Work out the finished part from the listing and answer in its coordinate system (mm). Face numbers are marked on the shaded views. A direction names the side the tool comes from. Give positions to 0.01 mm unless a question says otherwise; leave off trailing zeros. Loops run counter-clockwise (first coordinate to the right, second up) from the corner with the lowest first, then second, coordinate; pieces in that order, holes last. Notation, with made-up numbers: M 81.5,60 L 138.5,60 A25 cw 138.5,86 Z; hole C 64,8.5 d11. An arc over 180 degrees is marked long. Write item = value, one per line. Start each with the question number.
1. For the marked faces 1 and 2, determine the directions among +Z, -Z, +X, -X, +Y, -Y from which every point of the face is accessible in a straight line to the end or side of a thin tool.
2. Section B-B on z = -4.5 is taken. Determine the outline of the cut face in (x, y) (1 decimal), plus the area to 3 significant figures.
3. Flat-ended cylindrical pins translate along their axes: pin 1 Ø1 at (y, z) = (-2, -10) entering from -X; pin 2 Ø2 at (x, z) = (1, -9.5) entering from -Y; pin 3 Ø2 at (x, z) = (-2.5, -8) entering from -Y. Find the tip coordinate at first contact, or state that the pin passes through.
4. Section C-C on x = 2.75 is taken. Determine the outline of the cut face in (y, z) (3 decimals).
5. Consider L1, parallel to Z at x = 1.5, y = 2.5 (3 decimals); L2, parallel to Y at x = -1, z = -9.75; L3, parallel to Z at x = -0.75, y = -1 (3 decimals). Determine where each line is inside the solid, lowest interval first. Write a range as [from, to].
Solid Edge part; units mm, degrees
sketch "Sketch1" plane through (0, 0, 0) normal (0, 0, 1) x (1, 0, 0)
  circle A0 centre (0, 0) radius 6.4452
extrude "Protrusion1" add sketch "Sketch1" along normal blind 3.175
sketch "Sketch2" plane through (0, 0, 0) normal (0, 0, -1) x (1, 0, 0)
  circle A0 centre (0, 0) radius 2.0828
extrude "Protrusion2" add sketch "Sketch2" along normal blind 12.7
sketch "Sketch3" plane through (0, 0, -12.7) normal (0, 0, -1) x (1, 0, 0)
  circle A0 centre (0, 0) radius 2.0825
extrude "Cutout1" cut sketch "Sketch3" against normal blind 12.6873 flip side to cut
sketch "Sketch4" plane through (0, 0, 3.175) normal (0, 0, 1) x (1, 0, 0)
  line L0 (-5.609, 3.175) -> (5.609, 3.175)
extrude "Cutout2" cut sketch "Sketch4" against normal up to next material side at (0, 3.225, 3.175)
sketch "Sketch5" plane through (0, 0, 0) normal (1, 0, 0) x (0, 1, 0)
  line L0 (-0.7937, -12.7) -> (-2.0825, -10.4677)
revolve "RevolvedCutout1" cut sketch "Sketch5" angle 360 about axis through (0, 0, -14.7796) along (0, 0, 1) material side at (0, -1.4814, -11.6088)
pattern_circular "Pattern1" count 6 over 360 about axis through (0, 0, 3.175) along (0, 0, 1) of "Cutout2"
properties part number "24102273"
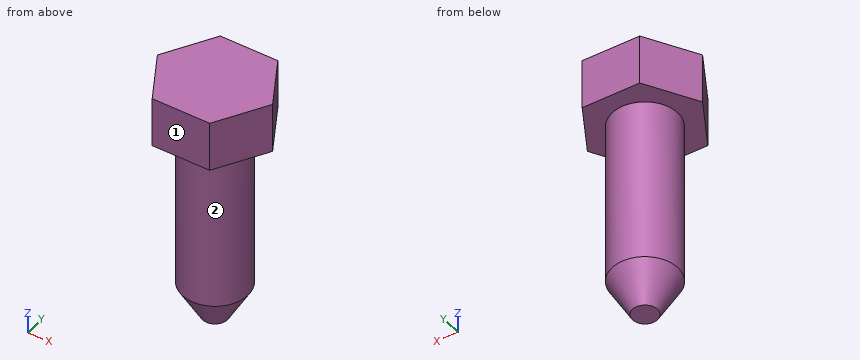
Verdict:
q1.face_1 = +Z, -Z, +X, -X, -Y
q1.face_2 = -Z
q2.outline = C 0,0 d4.2
q2.area = 13.6 mm2
q3.pin_1 = -1.44
q3.pin_2 = -2.08
q3.pin_3 = -1.44
q4.outline = M -1.587,0 L 1.587,0 L 1.587,3.175 L -1.587,3.175 Z
q5.L1 = [0, 3.175]
q5.L2 = [-1.83, 1.83]
q5.L3 = [-11.91, 3.175]
